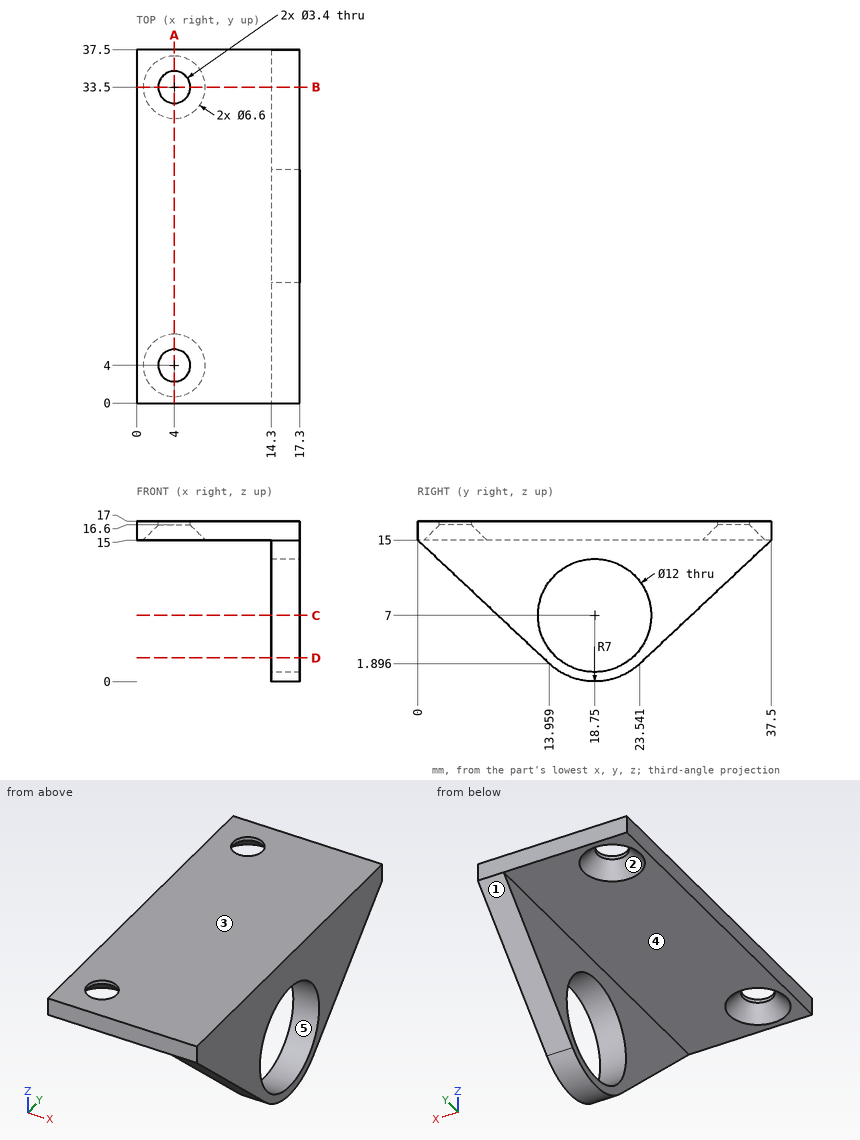
Job drawing, mm, ordinate dimensions from the low corner. One solid piece. A direction names the side the tool comes from. Round coordinates to 2 decimals unless told otherwise and drop trailing zeros. Loops run counter-clockwise (first coordinate to the right, second up) from the corner with the lowest first, then second, coordinate; pieces in that order, holes last.
(1) Cut at B-B (y = 33.5). Give the cut face in (x, z) (1 decimal), plus the area to 3 significant figures.
(2) Cut at C-C (z = 7). Give the cut face in (x, y).
(3) Which spindle directions (+Z, -Z, +X, -X, +Y, -Y) get a long thin tool onto all of the face, cutting with end or side? Do the marked faces 4 and 5. Say none if no direction does.
(4) Drop a flat-ended pin along its axis: pin 1 (1 mm diameter, centred on x = 11.5, y = 31, fed in from -Z). Give the stop position or say it passes through.
(5) Two-plate mould, pull along Y, no slides. Class the marked faces 1, 2 and 3: +Y half, -Y half, draft (parallel to the pull), parting line (faces both ways), or undercut.
(6) Cut at D-D (z = 2.5). Give the cut face in (x, y).
(7) Wall check: line 1 along Y through (x, z) = (4, 16.95); line 2 along X through (y, z) = (4, 16.8); line 3 along X through (y, z) = (10.5, 12.5). Give the ranges that are in metal, low to high.
(8) Cut at A-A (x = 4). Give the cut face in (y, z).
Findings below:
1. outline: (0, 15) - (0.7, 15) - (2.3, 16.6) - (2.3, 17) - (0, 17) - close; (5.7, 16.6) - (7.3, 15) - (14.3, 15) - (14.3, 11.2) - (17.3, 11.2) - (17.3, 17) - (5.7, 17) - close
1. area: 36.5 mm2
2. outline: (14.3, 8.52) - (17.3, 8.52) - (17.3, 12.75) - (14.3, 12.75) - close; (14.3, 24.75) - (17.3, 24.75) - (17.3, 28.98) - (14.3, 28.98) - close
3. face 4: -Z, -X, +Y, -Y
3. face 5: +X, -X
4. pin 1: stops at z = 15
5. face 1: +Y half
5. face 2: undercut
5. face 3: draft
6. outline: (14.3, 13.32) - (17.3, 13.32) - (17.3, 14.78) - (14.3, 14.78) - close; (14.3, 22.72) - (17.3, 22.72) - (17.3, 24.18) - (14.3, 24.18) - close
7. line 1: y = 0 to 2.3, 5.7 to 31.8, 35.2 to 37.5
7. line 2: x = 0 to 2.3, 5.7 to 17.3
7. line 3: x = 14.3 to 17.3
8. outline: (0, 15) - (0.7, 15) - (2.3, 16.6) - (2.3, 17) - (0, 17) - close; (5.7, 16.6) - (7.3, 15) - (30.2, 15) - (31.8, 16.6) - (31.8, 17) - (5.7, 17) - close; (35.2, 16.6) - (36.8, 15) - (37.5, 15) - (37.5, 17) - (35.2, 17) - close
